Verification items for the finished model (mm, model axes). A direction names the side the tool comes from. Give positions to 0.01 mm unless a question says otherwise; leave off trailing zeros. Write each loop counter-clockwise with the first axis right and the second up, starting at its lowest first coordinate (ties: lowest second). Pieces come first, ordered by that corner, then holes. Notation, with made-up numbers: (18.25, -6.5) -> (49.25, -6.5) arc R32 ccw to (49.25, 27.5) -> close; hole circle Ø9 at (-12.5, -14). An arc over 180 degrees is marked (long way). Write item = value, one per line.
from build123d import *

# Parameters (mm, degrees)
SKETCH_1_W           = 72.5
SKETCH_1_H           = 37
EXTRUDE_1_DEPTH      = 2
EXTRUDE_2_DEPTH      = 10
EXTRUDE_2_DEPTH_BACK = 2
SKETCH_3_R           = 1.65
EXTRUDE_3_DEPTH      = 2
FILLET_1_R           = 2
FILLET_2_R           = 1


with BuildPart() as part:
    # 草图1 → 凸台-拉伸1 (new body)
    with BuildSketch(Plane(origin=(0, 0, 0), x_dir=(1, 0, 0), z_dir=(0, 1, 0))):
        Rectangle(SKETCH_1_W, SKETCH_1_H)
    extrude(amount=EXTRUDE_1_DEPTH)

    # 草图2 → 凸台-拉伸2 (add, two sides: drawn at the far end of the back side and taken through both)
    with BuildSketch(Plane(origin=(0, 2, 0), x_dir=(1, 0, 0), z_dir=(0, 1, 0)).offset(-EXTRUDE_2_DEPTH_BACK)):
        Polygon((-36.25, 18.5), (-36.25, 14.5), (-39.25, 14.5), (-39.25, 21.5), (-32.25, 21.5), (-32.25, 18.5), align=None)
        Polygon((32.25, 18.5), (36.25, 18.5), (36.25, 14.5), (39.25, 14.5), (39.25, 21.5), (32.25, 21.5), align=None)
        Polygon((36.25, -18.5), (36.25, -14.5), (39.25, -14.5), (39.25, -21.5), (32.25, -21.5), (32.25, -18.5), align=None)
        Polygon((-32.25, -18.5), (-36.25, -18.5), (-36.25, -14.5), (-39.25, -14.5), (-39.25, -21.5), (-32.25, -21.5), align=None)
    extrude(amount=EXTRUDE_2_DEPTH + EXTRUDE_2_DEPTH_BACK)

    # 草图3 → 凸台-拉伸3 (add)
    # profile 1 of 4: a face of its own
    with BuildSketch(Plane(origin=(0, 2, 0), x_dir=(1, 0, 0), z_dir=(0, 1, 0))):
        with BuildLine():
            Line((25.25, 18.5), (25.25, 23.5))
            ThreePointArc((25.25, 23.5), (28.75, 27), (32.25, 23.5))
            Line((32.25, 23.5), (32.25, 18.5))
            Line((32.25, 18.5), (25.25, 18.5))
        make_face()
        with Locations(Location((28.75, 23.5, 0), (0, 0, 90))):
            Circle(SKETCH_3_R, mode=Mode.SUBTRACT)
    # profile 2 of 4: a face of its own
    with BuildSketch(Plane(origin=(0, 2, 0), x_dir=(1, 0, 0), z_dir=(0, 1, 0))):
        with BuildLine():
            Line((-32.25, 18.5), (-25.25, 18.5))
            Line((-25.25, 18.5), (-25.25, 23.5))
            ThreePointArc((-25.25, 23.5), (-28.75, 27), (-32.25, 23.5))
            Line((-32.25, 23.5), (-32.25, 18.5))
        make_face()
        with Locations(Location((-28.75, 23.5, 0), (0, 0, 270))):
            Circle(SKETCH_3_R, mode=Mode.SUBTRACT)
    # profile 3 of 4: a face of its own
    with BuildSketch(Plane(origin=(0, 2, 0), x_dir=(1, 0, 0), z_dir=(0, 1, 0))):
        with BuildLine():
            Line((32.25, -18.5), (25.25, -18.5))
            Line((25.25, -18.5), (25.25, -23.5))
            ThreePointArc((25.25, -23.5), (28.75, -27), (32.25, -23.5))
            Line((32.25, -23.5), (32.25, -18.5))
        make_face()
        with Locations(Location((28.75, -23.5, 0), (0, 0, 270))):
            Circle(SKETCH_3_R, mode=Mode.SUBTRACT)
    # profile 4 of 4: a face of its own
    with BuildSketch(Plane(origin=(0, 2, 0), x_dir=(1, 0, 0), z_dir=(0, 1, 0))):
        with BuildLine():
            Line((-25.25, -18.5), (-25.25, -23.5))
            ThreePointArc((-25.25, -23.5), (-28.75, -27), (-32.25, -23.5))
            Line((-32.25, -23.5), (-32.25, -18.5))
            Line((-32.25, -18.5), (-25.25, -18.5))
        make_face()
        with Locations(Location((-28.75, -23.5, 0), (0, 0, 90))):
            Circle(SKETCH_3_R, mode=Mode.SUBTRACT)
    extrude(amount=-EXTRUDE_3_DEPTH)

    # 圆角1
    fillet_1_edges = [part.edges().sort_by_distance(p)[0] for p in [
        (-25.25, 1, 18.5),
        (-36.25, 1, 14.5),
        (-36.25, 1, -14.5),
        (-25.25, 1, -18.5),
        (25.25, 1, -18.5),
        (36.25, 1, -14.5),
        (36.25, 1, 14.5),
        (-39.25, 6, 21.5),
        (39.25, 6, 21.5),
        (39.25, 6, -21.5),
        (-39.25, 6, -21.5),
        (-32.25, 1, -21.5),
        (32.25, 1, -21.5),
        (25.25, 1, 18.5),
        (32.25, 1, 21.5),
        (-32.25, 1, 21.5),
    ]]
    fillet(fillet_1_edges, radius=FILLET_1_R - 0.0001)  # a hair under: the kernel refuses the full size

    # 圆角2
    fillet_2_edges = [part.edges().sort_by_distance(p)[0] for p in [
        (-32.25, 2, 20),
        (32.25, 2, -20),
        (-36.25, 7, 18.5),
        (36.25, 7, 18.5),
        (36.25, 7, -18.5),
        (-36.25, 7, -18.5),
        (32.25, 2, 20),
        (-32.25, 2, -20),
    ]]
    fillet(fillet_2_edges, radius=FILLET_2_R)


solid = part.part
Item 1: Material ranges on line 1 (X direction, y = 0.4, z = -23.5); line 2 (Z direction, x = -30, y = 1.5), recorded low to high.
Response values:
line_1 = -32.25 to -30.4, -27.1 to -25.25, 25.25 to 27.1, 30.4 to 32.25
line_2 = -26.77 to -24.58, -22.42 to 22.42, 24.58 to 26.77
Item 2: Sectioned sample at C-C on z = -7.5. Record the cut outline in (x, y), then the cut area to 3 significant figures.
Response values:
outline = (-36.25, 0) -> (36.25, 0) -> (36.25, 2) -> (-36.25, 2) -> close
area = 145 mm^2
Item 3: Set-up check for faces 4 (the flat face through (34, 7, -18.5)), 5 (the flat face through (0, 1, -18.5)), 6 (the flat face through (0, 1, 18.5)): record each of +Z, -Z, +X, -X, +Y, -Y from which the full face is reachable in a straight line by a thin tool's end or side.
Response values:
face_4 = +Y
face_5 = -Z, +Y, -Y
face_6 = +Z, +Y, -Y
Item 4: Mould release check, pull along X, two halves, no side actions. Record for faces 1 (the cylindrical face through (29.865, 1.014, 22.284)), 2 (the cylindrical face through (-32.85, 1.01, 22.07)), 3 (the flat face through (1, 0, 0)): +X half, -X half, draft (parallel to the pull), parting line (faces both ways), or undercut.
Response values:
face_1 = undercut
face_2 = -X half
face_3 = draft
Item 5: Go/stop test with flat-tipped pins: P1, Ø6.5, axis at x = -34, y = 7, coming from the -Z side; P2, Ø5, axis at x = -35, y = 6.5, coming from the +Z side; P3, Ø5, axis at x = -20, z = 6, coming from the +Y side. Record where each tip stops, or that it passes through.
Response values:
P1 = -21.5
P2 = 21.5
P3 = 2
Item 6: Sectioned sample at B-B on x = -28.75. Record the cut outline in (y, z).
Response values:
outline = (0, -27) -> (2, -27) -> (2, -25.15) -> (0, -25.15) -> close; (0, -21.85) -> (2, -21.85) -> (2, 21.85) -> (0, 21.85) -> close; (0, 25.15) -> (2, 25.15) -> (2, 27) -> (0, 27) -> close
Item 7: Sectioned sample at D-D on x = -4. Record the cut outline in (y, z).
Response values:
outline = (0, -18.5) -> (2, -18.5) -> (2, 18.5) -> (0, 18.5) -> close
Item 8: Sectioned sample at A-A on y = 4. Give the number of separate pieces and of enclosed holes in the cut face, then the cut area to 3 significant figures.
Response values:
separate_pieces = 4
enclosed_holes = 0
area = 129 mm^2
